Part model, mm, in its own coordinate system. Round coordinates to 2 decimals unless told otherwise and drop trailing zeros. Loops run counter-clockwise (first coordinate to the right, second up) from the corner with the lowest first, then second, coordinate; pieces in that order, holes last. Notation, with made-up numbers: (-29.75, 11) - (21.25, 11) arc R21 ccw to (21.25, 32) - close; hole circle Ø10 at (24.25, 64). An arc over 180 degrees is marked (long way). Put each result on its own line as item: value.
from build123d import *

# Parameters (mm, degrees)
CROQUIS2_R = 1.25


with BuildPart() as part:
    # Barrer1: sweep along a path in Croquis1
    with BuildLine(Plane.XY) as barrer1_path:
        Line((-27.6, -5.9), (-25.75, -5.9))
        ThreePointArc((-25.75, -5.9), (-23.982233047, -5.167766953), (-23.25, -3.4))
        Line((-23.25, -3.4), (-23.25, -2.5))
        ThreePointArc((-23.25, -2.5), (-22.517766953, -0.732233047), (-20.75, 0))
        Line((-20.75, 0), (20.75, 0))
        ThreePointArc((20.75, 0), (22.517766953, -0.732233047), (23.25, -2.5))
        Line((23.25, -2.5), (23.25, -3.4))
        ThreePointArc((23.25, -3.4), (23.982233047, -5.167766953), (25.75, -5.9))
        Line((25.75, -5.9), (27.6, -5.9))
    # Croquis2 → Barrer1 (sweep)
    with BuildSketch(Plane(origin=(27.6, 0, 0), x_dir=(0, 0, -1), z_dir=(1, 0, 0))):
        with Locations((0, -5.9)):
            Circle(CROQUIS2_R)
    sweep(path=barrer1_path.line)


solid = part.part
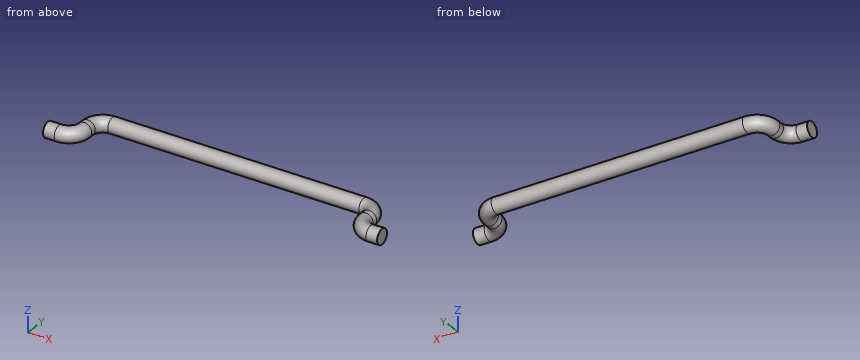
1. Pin check, flat tip, straight feed: P1, Ø1, axis at y = -3, z = 0, coming from the +X side. Stop position of the tip, or through.
A:
P1: stops at x = 24.5
2. Band-saw the part on A-A (z = 0). List the corners of the cut face in (x, y), plus the area to 3 significant figures.
A:
outline: (-27.6, -7.15) - (-25.75, -7.15) arc R3.75 ccw to (-22, -3.4) - (-22, -2.5) arc R1.25 cw to (-20.75, -1.25) - (20.75, -1.25) arc R1.25 cw to (22, -2.5) - (22, -3.4) arc R3.75 ccw to (25.75, -7.15) - (27.6, -7.15) - (27.6, -4.65) - (25.75, -4.65) arc R1.25 cw to (24.5, -3.4) - (24.5, -2.5) arc R3.75 ccw to (20.75, 1.25) - (-20.75, 1.25) arc R3.75 ccw to (-24.5, -2.5) - (-24.5, -3.4) arc R1.25 cw to (-25.75, -4.65) - (-27.6, -4.65) - close
area: 157 mm²
3. Probe line 1 along X through (y, z) = (-2, 0.95); line 2 along Y through (x, z) = (-20.5, 0.05); line 3 along X through (y, z) = (-4, 0.2). List the from-to ranges inside material, lowest first. Write a range as [from, to].
A:
line 1: x = [-24.02, -22.36], [22.36, 24.02]
line 2: y = [-1.25, 1.25]
line 3: x = [-24.64, -22.06], [22.06, 24.64]
